Solid Edge part; units mm, degrees
sketch "Sketch1" plane through (0, 0, 0) normal (0, -1, 0) x (1, 0, 0)
  line L0 (0, 0) -> (14, 0)
  line L1 (14, 0) -> (14, 5)
  line L2 (50, 5) -> (14, 5)
  line L3 (50, 19) -> (50, 5)
  line L4 (14, 19) -> (50, 19)
  line L5 (14, 19) -> (0, 19)
  line L6 (0, 19) -> (0, 0)
  dimension "D1" = 50
  dimension "D2" = 50
  dimension "D3" = 14
extrude "Protrusion1" add sketch "Sketch1" along normal mid plane 58
sketch "Sketch2" plane through (0, 0, 10.5) normal (-1, 0, 0) x (0, -1, 0)
  circle A0 centre (-22, 2.5) radius 3.2
  dimension "D1" = 22
extrude "Cutout1" cut sketch "Sketch2" against normal through all
mirror "Mirror1" about plane through (0, 0, 0) normal (0, -1, 0) of "Cutout1"
sketch "Sketch3" plane through (27, -29, 10.5) normal (0, -1, 0) x (0, 0, 1)
  circle A0 centre (-3.5, 20) radius 3.2
  dimension "D1" = 3.5
extrude "Cutout2" cut sketch "Sketch3" against normal through all
sketch "Sketch4" plane through (32, 0, 5) normal (0, 0, -1) x (-1, 0, 0)
  circle A0 centre (-0.4, 0) radius 13
extrude "Cutout3" cut sketch "Sketch4" against normal through all
sketch "Sketch5" plane through (32, 0, 10) normal (0, 0, -1) x (0, -1, 0)
  line L0 (17.4, 12.6) -> (17.4, -22.4304)
  line L1 (-13, 17) -> (13, 17)
  line L2 (-17.4, 12.6) -> (-17.4, -23.1466)
  arc A0 (-13, 17) -> (-17.4, 12.6) centre (-13, 12.6) ccw
  arc A1 (17.4, 12.6) -> (13, 17) centre (13, 12.6) ccw
extrude "Cutout4" cut sketch "Sketch5" along normal through all material side at (36.9152, -17.35, 10)
sketch "Sketch6" plane through (0, 0, 10.5) normal (-1, 0, 0) x (0, 1, 0)
  line L0 (-22, -2.5) -> (-19.6981, -0.2771)
  line L1 (-19.6981, -0.2771) -> (-22, 2.1066)
  line L2 (-22, 2.1066) -> (-24.3019, -0.2771)
  line L3 (-24.3019, -0.2771) -> (-22, -2.5)
extrude "Cutout5" cut sketch "Sketch6" against normal through all
mirror "Mirror2" about plane through (0, 0, 0) normal (0, -1, 0) of "Cutout5"
sketch "Sketch7" plane through (25, 29, 10.5) normal (0, 1, 0) x (1, 0, 0)
  line L0 (-18, 3.5) -> (-15.6981, 5.7229)
  line L1 (-15.6981, 5.7229) -> (-18, 8.1066)
  line L2 (-18, 8.1066) -> (-20.3019, 5.7229)
  line L3 (-20.3019, 5.7229) -> (-18, 3.5)
extrude "Cutout7" cut sketch "Sketch7" against normal through all
sketch "Sketch8" plane through (32.5, 0, 10) normal (0, 0, -1) x (0, 1, 0)
  circle A0 centre (-13, 12.9) radius 1.7
  circle A1 centre (13, 12.9) radius 1.7
  circle A2 centre (13, -13.1) radius 1.7
  circle A3 centre (-13, -13.1) radius 1.7
extrude "Cutout8" cut sketch "Sketch8" against normal through all
Check sheet for the modelled part. Datum: model origin and axes. Units: mm. A direction names the side the tool comes from. Give positions to 0.01 mm unless a question says otherwise; leave off trailing zeros. Loops run counter-clockwise (first coordinate to the right, second up) from the corner with the lowest first, then second, coordinate; pieces in that order, holes last. Notation, with made-up numbers: (66.25, -40) - (110.25, -40) arc R10 cw to (110.25, -21) - close; hole circle Ø6 at (-4.75, 31.25). An arc over 180 degrees is marked (long way). One line per question, with ' | ' between items. Start each with the question number.
1. Gauge pin test, flat ends, axial feed: pin 1 Ø1.5 at (x, y) = (39, 8) entering from +Z; pin 2 Ø4 at (x, y) = (45.4, -13) entering from -Z; pin 3 Ø1.5 at (y, z) = (13, 1.5) entering from +X. Record the tip position at first contact, or that the pin passes through.
2. Cross-section at D-D, the plane z = 7. Enter the section's corners in (x, y).
3. Material ranges on line 1 along Y through (x, z) = (14.5, 13); line 2 along Y through (x, z) = (22, 12); line 3 along Z through (x, y) = (4.5, -24.5), recorded low to high. Write a range as [from, to].
4. Cross-section at A-A, the plane y = 5. Give the number of separate pieces and of enclosed holes in the cut face, plus the area to 3 significant figures.
5. Draft check along X on faces 1 (the flat face through (8.167, 0.406, 3.602)), 2 (the cylindrical face through (24.6, 21.9, 16.2)), 3 (the flat face through (14, 0, 2)). Enter one of: released by +X, released by -X, zero draft, split by the parting line, or undercut.
6. Set-up check for faces 4 (the flat face through (0, 0, 10)), 5 (the flat face through (24.65, 23.167, 9.602)), 6 (the flat face through (15, 0, 8)): record each of +Z, -Z, +X, -X, +Y, -Y from which the full face is reachable in a straight line by a thin tool's end or side.
7. Cross-section at B-B, the plane z = 13. Enter the section's corners in (x, y).
Check result:
1) pin 1: passes through | pin 2: stops at z = 10 | pin 3: stops at x = 14
2) outline: (0, -29) - (3.8, -29) - (3.8, 29) - (0, 29) - close; (10.2, -29) - (50, -29) - (50, -17.4) - (19.4, -17.4) arc R4.4 cw to (15, -13) - (15, 13) arc R4.4 cw to (19.4, 17.4) - (50, 17.4) - (50, 29) - (10.2, 29) - close
3) line 1: y = [-29, -25.2], [-18.8, 18.8], [25.2, 29] | line 2: y = [-29, -25.04], [-18.96, -7.8], [7.8, 18.96], [25.04, 29] | line 3: z = [0, 5], [9, 11], [15, 19]
4) separate pieces: 2 | enclosed holes: 1 | area: 344 mm2
5) face 1: undercut | face 2: zero draft | face 3: released by +X
6) face 4: +Z, -Z, -X, +Y, -Y | face 5: +X, -X | face 6: -Z, +X
7) outline: (0, -29) - (50, -29) - (50, -25.2) - (0, -25.2) - close; (0, -18.8) - (50, -18.8) - (50, 18.8) - (0, 18.8) - close; (0, 25.2) - (50, 25.2) - (50, 29) - (0, 29) - close; hole circle Ø3.4 at (19.4, -13); hole circle Ø3.4 at (19.4, 13); hole circle Ø26 at (32.4, 0); hole circle Ø3.4 at (45.4, -13); hole circle Ø3.4 at (45.4, 13)
